from build123d import *

# Parameters (mm, degrees)
F0_R     = 32.717526
F1_DEPTH = 6.35
F2_SIZE  = 5.08
F3_R     = 32.935812
F4_DEPTH = 76.2
F5_R     = 33.341524
F6_DEPTH = 6.35
F7_SIZE  = 5.08


with BuildPart() as f1:
    # F0 (on Top) → F1 (new body)
    with BuildSketch(Plane.XY):
        Circle(F0_R)
    extrude(amount=F1_DEPTH)

    # F2
    f2_edges = [f1.edges().sort_by_distance(p)[0] for p in [
        (-32.717526, 0, 6.35),
    ]]
    chamfer(f2_edges, length=F2_SIZE)

    # F3 (on face) → F4 (join)
    with BuildSketch(Plane(origin=(0, 0, 0), x_dir=(1, 0, 0), z_dir=(0, 0, -1))):
        Circle(F3_R)
    extrude(amount=F4_DEPTH)

    # F5 (on face) → F6 (join)
    with BuildSketch(Plane(origin=(0, 0, -76.2), x_dir=(1, 0, 0), z_dir=(0, 0, -1))):
        Circle(F5_R)
    extrude(amount=F6_DEPTH)

    # F7
    f7_edges = [f1.edges().sort_by_distance(p)[0] for p in [
        (-33.341524, 0, -82.55),
    ]]
    chamfer(f7_edges, length=F7_SIZE)


solid = f1.part
Geometry: final body of the model. Coordinates: model frame, mm. A direction names the side the tool comes from. Round coordinates to 2 decimals unless told otherwise and drop trailing zeros. Order: outer loops, then holes, each group sorted by start corner. A loop starts at its lowest first (then second) coordinate and runs counter-clockwise, first axis right, second up.
Q1. Section C-C, the plane z = -40. Output: boundary loops of the cut face in (x, y), and give its area (3 significant figures).
Result sheet:
outline: circle Ø65.87 at (0, 0)
area: 3,410 mm2
Q2. Material intervals for probe 1 along Y at (x, z) = (-0.5, -10); probe 2 along X at (y, z) = (19, -65); probe 3 along Y at (x, z) = (11, -54.5), sorted ascending.
Result sheet:
probe 1: y = -32.93 to 32.93
probe 2: x = -26.9 to 26.9
probe 3: y = -31.04 to 31.04
Q3. Section A-A, the plane y = 0. Output: boundary loops of the cut face in (x, z).
Result sheet:
outline: (-33.34, -77.47) - (-28.26, -82.55) - (28.26, -82.55) - (33.34, -77.47) - (33.34, -76.2) - (32.94, -76.2) - (32.94, 0) - (32.72, 0) - (32.72, 1.27) - (27.64, 6.35) - (-27.64, 6.35) - (-32.72, 1.27) - (-32.72, 0) - (-32.94, 0) - (-32.94, -76.2) - (-33.34, -76.2) - close
Q4. Access query for faces 1 (the face through (31.207, 9.827, 0.626)), 2 (the face through (-33.31, -1.47, -76.83)). Directions: +Z, -Z, +X, -X, +Y, -Y. A direction counts if a zero-diameter tool reaches every point of the face in a straight line with its end or side. Return the directions, or none.
Result sheet:
face 1: +Z
face 2: +Z, -Z
Q5. Pin query (flat end, axial travel): pin 1 (8 mm diameter, centred on y = -19, z = -34, fed in from +X); pin 2 (2 mm diameter, centred on x = -5, z = -18.5, fed in from -Y); pin 3 (8 mm diameter, centred on x = 25.5, y = -26, fed in from -Z); pin 4 (5 mm diameter, centred on x = -26, y = 15, fed in from -Z). Return the tip coordinate at first contact, or that it passes through.
Result sheet:
pin 1: stops at x = 29.32
pin 2: stops at y = -32.69
pin 3: stops at z = -78.39
pin 4: stops at z = -82.55
